from build123d import *

# Parameters (mm, degrees)
SKETCH1_W                      = 12.75
SKETCH1_H                      = 12.5
BOSS_EXTRUDE1_DEPTH            = 10.24
BOSS_EXTRUDE2_DEPTH            = 0.3
F_15_0_15_DIAMETER_HOLE1_D     = 15
F_15_0_15_DIAMETER_HOLE1_DEPTH = 23.04
CHAMFER1_SIZE                  = 2


with BuildPart() as part:
    # Sketch1 → Revolve1 (revolve)
    with BuildSketch(Plane.XY, mode=Mode.PRIVATE) as revolve1_sk:
        with Locations((6.375, 18.15)):
            Rectangle(SKETCH1_W, SKETCH1_H)
    revolve(revolve1_sk.sketch.rotate(Axis((0, 24.4, 0), (0, -1, 0)), 270), axis=Axis((0, 24.4, 0), (0, -1, 0)))

    # Sketch2 → Boss-Extrude1 (add)
    with BuildSketch(Plane(origin=(0, 24.4, 0), x_dir=(-1, 0, 0), z_dir=(0, 1, 0))):
        with BuildLine():
            Line((2.9, -11.90178558), (2.9, -11.975))
            ThreePointArc((2.9, -11.975), (0, -14.875), (-2.9, -11.975))
            Line((-2.9, -11.975), (-2.9, -11.90178558))
            ThreePointArc((-2.9, -11.90178558), (0, 12.25), (2.9, -11.90178558))
        make_face()
    extrude(amount=BOSS_EXTRUDE1_DEPTH)

    # Sketch3 → Boss-Extrude2 (add)
    with BuildSketch(Plane(origin=(0, 34.64, 0), x_dir=(-1, 0, 0), z_dir=(0, 1, 0))):
        with BuildLine():
            Line((1, -8.975), (1, -11.975))
            ThreePointArc((1, -11.975), (0, -12.975), (-1, -11.975))
            Line((-1, -11.975), (-1, -8.975))
            ThreePointArc((-1, -8.975), (0, -7.975), (1, -8.975))
        make_face()
    extrude(amount=BOSS_EXTRUDE2_DEPTH)

    # Ø15.0 (15) Diameter Hole1
    with Locations(Plane(origin=(0, 11.9, 0), x_dir=(-1, 0, 0), z_dir=(0, -1, 0))):
        with Locations((0, 0)):
            Hole(F_15_0_15_DIAMETER_HOLE1_D / 2, depth=F_15_0_15_DIAMETER_HOLE1_DEPTH)

    # Chamfer1
    chamfer1_edges = [part.edges().sort_by_distance(p)[0] for p in [
        (0, 34.64, 12.25),
    ]]
    chamfer(chamfer1_edges, length=CHAMFER1_SIZE)


solid = part.part
Verification items for the finished model (mm, model axes). A direction names the side the tool comes from. Give positions to 0.01 mm unless a question says otherwise; leave off trailing zeros. Write each loop counter-clockwise with the first axis right and the second up, starting at its lowest first coordinate (ties: lowest second). Pieces come first, ordered by that corner, then holes. Notation, with made-up numbers: (62, 56) -> (93, 56) arc R25 ccw to (93, 78) -> close; hole circle Ø9 at (-7.75, 46.25). An arc over 180 degrees is marked (long way). Use CSV: the item, a comma, the result in double quotes.
(1) Sectioned sample at D-D (y = 18). Record the cut outline in (x, z), plus the area to 3 significant figures.
Derived:
outline,"circle Ø25.5 at (0, 0); hole circle Ø15 at (0, 0)"
area,"334 mm^2"
(2) Sectioned sample at B-B (x = 0). Record the cut outline in (y, z) (3 decimals).
Derived:
outline,"(11.9, -12.75) -> (24.4, -12.75) -> (24.4, -14.875) -> (34.64, -14.875) -> (34.64, -12.975) -> (34.94, -12.975) -> (34.94, -7.975) -> (34.64, -7.975) -> (34.64, -7.5) -> (11.9, -7.5) -> close; (11.9, 7.5) -> (34.64, 7.5) -> (34.64, 10.25) -> (32.64, 12.25) -> (24.4, 12.25) -> (24.4, 12.75) -> (11.9, 12.75) -> close"
(3) Sectioned sample at C-C (y = 31). Record the cut outline in (x, z) (3 decimals).
Derived:
outline,"(-2.9, -11.975) arc R2.9 ccw to (2.9, -11.975) -> (2.9, -11.902) arc R12.25 ccw (long way) to (-2.9, -11.902) -> close; hole circle Ø15 at (0, 0)"
(4) Go/stop test with flat-tipped pins: pin 1 (6 mm diameter, centred on x = 4, z = -3.5, fed in from +Y); pin 2 (1.5 mm diameter, centred on y = 22.5, z = 9.5, fed in from +X); pin 3 (1.7 mm diameter, centred on y = 28.5, z = -10.5, fed in from +X); pin 4 (2.5 mm diameter, centred on x = 0, z = -13.5, fed in from -Y). Record where each tip stops, or that it passes through.
Derived:
pin 1,"stops at y = 34.64"
pin 2,"stops at x = 9.27"
pin 3,"stops at x = 7.55"
pin 4,"stops at y = 11.9"
(5) Release check for a two-part mould opening along X. For faces 1 (the cylindrical face through (-7.493, 23.429, -0.33)), 2 (the conical face through (0.43, 34.32, 10.56)), 3 (the flat face through (-0.1, 34.64, -7.7)) record: +X half, -X half, draft (parallel to the pull), parting line (faces both ways), or undercut.
Derived:
face 1,"undercut"
face 2,"parting line"
face 3,"draft"
(6) Sectioned sample at A-A (z = 0). Record the cut outline in (x, y), plus the area to 3 significant figures.
Derived:
outline,"(-12.75, 11.9) -> (-7.5, 11.9) -> (-7.5, 34.64) -> (-10.25, 34.64) -> (-12.25, 32.64) -> (-12.25, 24.4) -> (-12.75, 24.4) -> close; (7.5, 11.9) -> (12.75, 11.9) -> (12.75, 24.4) -> (12.25, 24.4) -> (12.25, 32.64) -> (10.25, 34.64) -> (7.5, 34.64) -> close"
area,"225 mm^2"
(7) Material ranges on L1, parallel to Z at x = 0, y = 18; L2, parallel to Y at x = 5, z = -7; L3, parallel to Z at x = 6.75, y = 29.25, recorded low to high.
Derived:
L1,"z = -12.75 to -7.5, 7.5 to 12.75"
L2,"y = 11.9 to 34.64"
L3,"z = -10.22 to -3.27, 3.27 to 10.22"
(8) Set-up check for faces 4 (the flat face through (2.9, 33.3, -11.5)), 5 (the cylindrical face through (0.5, 28.46, 12.24)), 6 (the flat face through (-2.9, 33.3, -11.5)): record each of +Z, -Z, +X, -X, +Y, -Y from which the full face is reachable in a straight line by a thin tool's end or side.
Derived:
face 4,"-Z, +X, +Y"
face 5,"+Y"
face 6,"-Z, -X, +Y"
